Answer from the drawing. Dimensions are ordinates in mm from the lowest x, y and z of the part. A direction names the side the tool comes from. Give positions to 0.01 mm unless a question says otherwise; leave off trailing zeros. Order: outer loops, then holes, each group sorted by start corner. A loop starts at its lowest first (then second) coordinate and runs counter-clockwise, first axis right, second up.
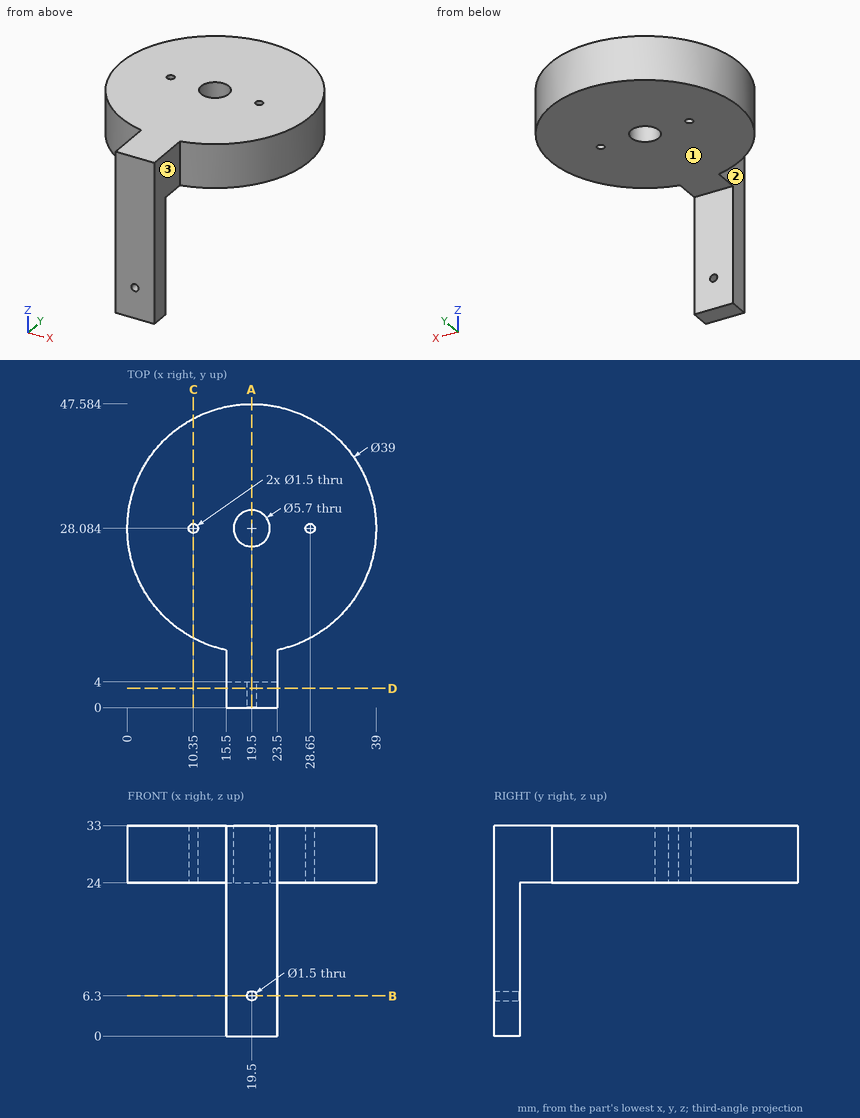
1. The part is cut by section D-D (y = 3). Write down the section's boundary in (x, z).
Findings below:
outline: (15.5, 0) - (23.5, 0) - (23.5, 33) - (15.5, 33) - close; hole circle Ø1.5 at (19.5, 6.3)
2. Which of the six approach directions +Z, -Z, +X, -X, +Y, -Y give full straight-line access (tool end or side, diameter ignored) to the marked faces 1, 2 and 3?
Findings below:
face 1: -Z, +X, -X, +Y
face 2: +Z, -Z, -X, -Y
face 3: +Z, -Z, +X, -Y
3. The part is cut by section A-A (x = 19.5). Write down the section's boundary in (y, z), then the cut area to 3 significant figures.
Findings below:
outline: (0, 0) - (4, 0) - (4, 5.55) - (0, 5.55) - close; (0, 7.05) - (4, 7.05) - (4, 24) - (25.23, 24) - (25.23, 33) - (0, 33) - close; (30.93, 24) - (47.58, 24) - (47.58, 33) - (30.93, 33) - close
area: 467 mm2
4. Straight lines are drawn through the part: probe 1 along Y at (x, z) = (19.5, 27.25); probe 2 along Z at (x, y) = (19.5, 13); probe 3 along X at (y, z) = (6.5, 25). For each, find the intervals that lie inside material, in ascending order.
Findings below:
probe 1: y = 0 to 25.23, 30.93 to 47.58
probe 2: z = 24 to 33
probe 3: x = 15.5 to 23.5
5. The part is cut by section B-B (z = 6.3). Write down the section's boundary in (x, y), then the cut area to 3 significant figures.
Findings below:
outline: (15.5, 0) - (18.75, 0) - (18.75, 4) - (15.5, 4) - close; (20.25, 0) - (23.5, 0) - (23.5, 4) - (20.25, 4) - close
area: 26.0 mm2
6. The part is cut by section C-C (x = 10.35). Write down the section's boundary in (y, z), then the cut area to 3 significant figures.
Findings below:
outline: (10.86, 24) - (27.33, 24) - (27.33, 33) - (10.86, 33) - close; (28.83, 24) - (45.3, 24) - (45.3, 33) - (28.83, 33) - close
area: 296 mm2
7. Given P1, Ø1.4, axis at x = 10.35, y = 28.08, coming from the -Z side; P2, Ø19.5, axis at x = 26, y = 29, coming from the -Z side; P3, Ø2.5, axis at y = 3.5, z = 23.5, coming from the -X side; P4, Ø4.5, axis at y = 5.5, z = 10, coming from the +X side, each flat-ended and moving along its own axis, determine where each tip first touches the part or whether it passes through.
Findings below:
P1: passes through
P2: stops at z = 24
P3: stops at x = 15.5
P4: stops at x = 23.5
